Source: three-view drawing plus pictorial views. Frame: mm from the lowest corner of the part. A direction names the side the tool comes from. Coordinates: 2 decimals unless noted, no trailing zeros. Loops run counter-clockwise (first coordinate to the right, second up) from the corner with the lowest first, then second, coordinate; pieces in that order, holes last. Notation, with made-up numbers: (12.25, 62) - (58.25, 62) arc R13 ccw to (58.25, 82) - close; hole circle Ø2 at (38, -20.5). An arc over 180 degrees is marked (long way). Use CSV: the item, a comma, the result in double quotes. Start each with the question number.
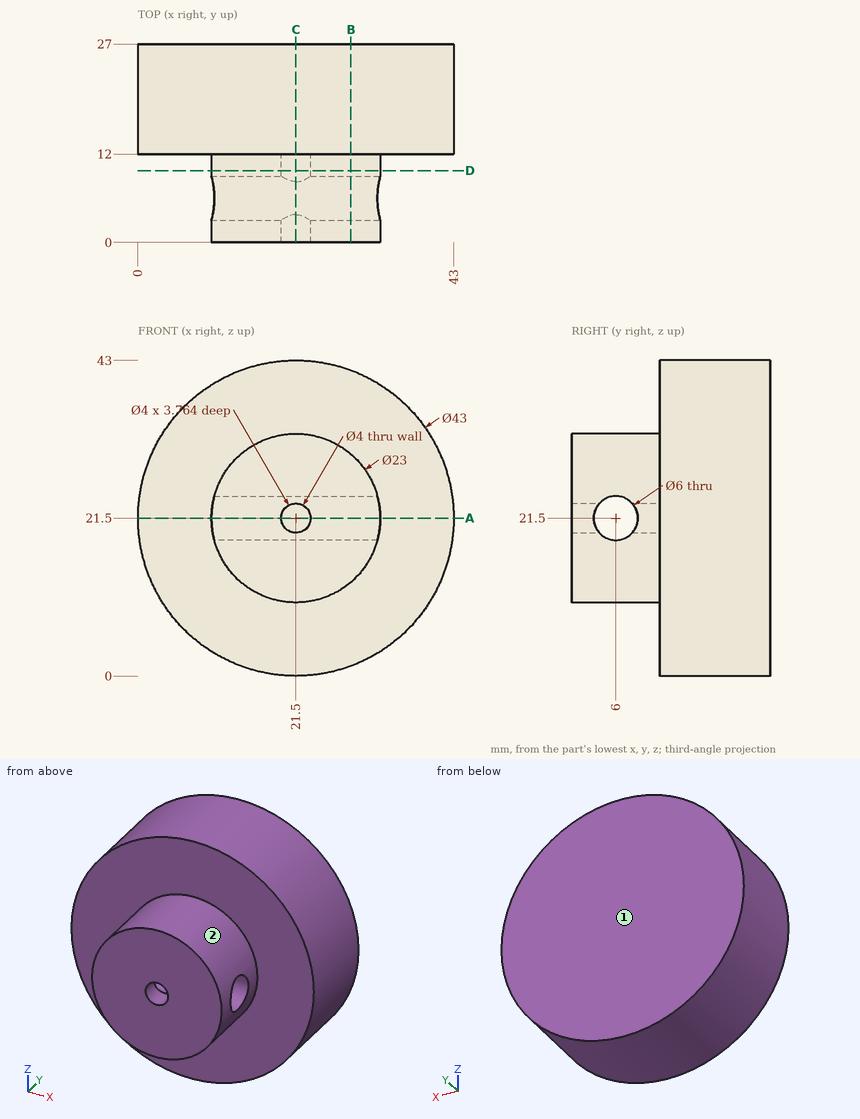
(1) Reachability of the marked faces 1 and 2 from +Z, -Z, +X, -X, +Y, -Y: full face, straight path, thin tool, end or side. Return the list, or none.
(2) Section D-D on y = 9.75. Output: boundary loops of the cut face in (x, z), plus the area to 3 significant figures.
(3) Ray query, line 1 (Z direction, x = 21.5, y = 2.8); line 2 (Y direction, x = 28, z = 21.5). Return the intervals inside material, ascending. Write a range as [from, to].
(4) Pin query (flat end, axial travel): pin 1 Ø5 at (x, z) = (6, 31.5) entering from -Y; pin 2 Ø6 at (y, z) = (14.5, 20) entering from -X; pin 3 Ø5.5 at (y, z) = (6, 21.5) entering from +X; pin 4 Ø1 at (y, z) = (12, 4.5) entering from -X. Return the tip coordinate at first contact, or that it passes through.
(5) Section B-B on x = 29. Output: boundary loops of the cut face in (y, z).
(6) Section A-A on z = 21.5. Output: boundary loops of the cut face in (x, y), plus the area to 3 significant figures.
(7) Section C-C on x = 21.5. Output: boundary loops of the cut face in (y, z), plus the area to 3 significant figures.
Solution:
1,face 1,"+Z, -Z, +X, -X, +Y"
1,face 2,"-Y"
2,outline,"circle Ø23 at (21.5, 21.5); hole circle Ø4 at (21.5, 21.5)"
2,area,"403 mm²"
3,line 1,"z = [10, 19.5], [23.5, 33]"
3,line 2,"y = [0, 3], [9, 27]"
4,pin 1,"stops at y = 12"
4,pin 2,"stops at x = 0"
4,pin 3,"passes through"
4,pin 4,"stops at x = 7.72"
5,outline,"(0, 12.78) - (12, 12.78) - (12, 1.35) - (27, 1.35) - (27, 41.65) - (12, 41.65) - (12, 30.22) - (0, 30.22) - close; hole circle Ø6 at (6, 21.5)"
6,outline,"(0, 12) - (10, 12) - (10, 9) - (19.5, 9) - (19.5, 12) - (23.5, 12) - (23.5, 9) - (33, 9) - (33, 12) - (43, 12) - (43, 27) - (0, 27) - close; (10, 0) - (19.5, 0) - (19.5, 3) - (10, 3) - close; (23.5, 0) - (33, 0) - (33, 3) - (23.5, 3) - close"
6,area,"759 mm²"
7,outline,"(0, 10) - (12, 10) - (12, 0) - (27, 0) - (27, 43) - (12, 43) - (12, 33) - (0, 33) - (0, 23.5) - (3.76, 23.5) arc R3 cw to (8.24, 23.5) - (12, 23.5) - (12, 19.5) - (8.24, 19.5) arc R3 cw to (3.76, 19.5) - (0, 19.5) - close"
7,area,"867 mm²"
